Geometry check sheet. Reference: the model listing, model coordinates, mm. Give positions to 0.01 mm unless a question says otherwise; leave off trailing zeros. Write each loop counter-clockwise with the first axis right and the second up, starting at its lowest first coordinate (ties: lowest second). Pieces come first, ordered by that corner, then holes. Notation, with made-up numbers: (89.5, -28.5) -> (119.5, -28.5) arc R22 ccw to (119.5, 5.5) -> close; hole circle Ø6 at (-10.75, 33). An arc over 180 degrees is marked (long way). Use a Markdown table: item, result. Add a question column.
from build123d import *

# Parameters (mm, degrees)
CYLINDER_R     = 16
CYLINDER_DEPTH = 120
PAD_DEPTH      = 100


with BuildPart() as cylinder:
    # Cylinder → Cylinder (new body)
    with BuildSketch(Plane.XY):
        Circle(CYLINDER_R)
    extrude(amount=CYLINDER_DEPTH)


with BuildPart() as cut:
    # Sketch → Pad (new body)
    with BuildSketch(Plane.XY):
        Polygon((400, -165.685425), (400, 165.685425), (165.685425, 400), (-165.685425, 400), (-400, 165.685425), (-400, -165.685425), (-165.685425, -400), (165.685425, -400), align=None)
    extrude(amount=PAD_DEPTH)

    # Cut: cut Cylinder
    add(cylinder.part, mode=Mode.SUBTRACT)


solid = cut.part
1) Sectioned sample at A-A, the plane y = 0. Enter the section's corners in (x, z), and give its area (3 significant figures).
2) Sectioned sample at B-B, the plane z = 88. Enter the section's corners in (x, y).
3) Sectioned sample at D-D, the plane x = -188. Enter the section's corners in (y, z).
4) Material ranges on probe 1 along Y at (x, z) = (0, 45.5); probe 2 along Y at (x, z) = (173, 56), recorded low to high. Write a range as [from, to].
5) Gauge pin test, flat ends, axial feed: P1, Ø2, axis at y = 171.5, z = 35, coming from the +X side; P2, Ø2, axis at y = 199, z = 87, coming from the -X side. Record the tip position at first contact, or that the pin passes through.
Check values:
| question | item | result |
|---|---|---|
| 1 | outline | (-400, 0) -> (-16, 0) -> (-16, 100) -> (-400, 100) -> close; (16, 0) -> (400, 0) -> (400, 100) -> (16, 100) -> close |
| 1 | area | 76,800 mm² |
| 2 | outline | (-400, -165.69) -> (-165.69, -400) -> (165.69, -400) -> (400, -165.69) -> (400, 165.69) -> (165.69, 400) -> (-165.69, 400) -> (-400, 165.69) -> close; hole circle Ø32 at (0, 0) |
| 3 | outline | (-377.69, 0) -> (377.69, 0) -> (377.69, 100) -> (-377.69, 100) -> close |
| 4 | probe 1 | [-400, -16], [16, 400] |
| 4 | probe 2 | [-392.69, 392.69] |
| 5 | P1 | x = 395.19 |
| 5 | P2 | x = -367.69 |
